Input: part model. Units: mm. Frame: model coordinates. A direction names the side the tool comes from. Give positions to 0.01 mm unless a question says otherwise; leave off trailing zeros. Order: outer loops, then holes, each group sorted by start corner. A loop starts at its lowest first (then second) coordinate and runs counter-clockwise, first axis right, second up. Notation, with made-up numbers: (9.5, -29.75) -> (46.5, -29.75) arc R23 ccw to (46.5, -10.75) -> close; hole circle Ø8 at (43.25, -28.5). An arc over 180 degrees is marked (long way). Use a Markdown table: item, result. Add a question column.
from build123d import *

# Parameters (mm, degrees)
SKETCH1_R                                    = 5
SKETCH1_R_2                                  = 2.5
BOSS_EXTRUDE1_DEPTH                          = 23.5
CSK_FOR_M5_COUNTERSUNK_FLAT_HEAD_SCR_2_COUNT = 2
CSK_FOR_M5_COUNTERSUNK_FLAT_HEAD_SCR_2_PITCH = 25
CUT_EXTRUDE1_DEPTH                           = 31.020826105
CUT_EXTRUDE1_DEPTH_BACK                      = 31.020826105
SKETCH4_W                                    = 10
SKETCH4_H                                    = 11.75


with BuildPart() as part:
    # Sketch1 → Boss-Extrude1 (new, symmetric)
    # profile 1 of 2: a face of its own
    with BuildSketch(Plane.XY):
        with BuildLine():
            Line((-18, -5), (0, -5))
            ThreePointArc((0, -5), (-2.958039892, -4.031128874), (-4.769696007, -1.5))
            Line((-4.769696007, -1.5), (-18, -1.5))
            Line((-18, -1.5), (-18, -5))
        make_face()
    # profile 2 of 2: a face of its own
    with BuildSketch(Plane.XY):
        Circle(SKETCH1_R)
        Circle(SKETCH1_R_2, mode=Mode.SUBTRACT)
    extrude(amount=BOSS_EXTRUDE1_DEPTH, both=True)

    # Sketch3 → CSK for M5 Countersunk Flat Head Screw1 (revolve, cut)
    with BuildSketch(Plane(origin=(-10.5, -1.5, -12.5), x_dir=(0, 0, 1), z_dir=(1, 0, 0))):
        Polygon((0, 0), (0, 3.5), (2.75, 3.5), (2.75, 2.45), (5.2, 0), align=None)
    csk_for_m5_countersunk_flat_head_screw1 = revolve(axis=Axis((-10.5, 4.85, -12.5), (0, -1, 0)), mode=Mode.SUBTRACT)

    # CSK for M5 Countersunk Flat Head Scr 2: CSK for M5 Countersunk Flat Head Screw1 ×2
    with Locations(*[(0, 0, i * CSK_FOR_M5_COUNTERSUNK_FLAT_HEAD_SCR_2_PITCH) for i in range(1, CSK_FOR_M5_COUNTERSUNK_FLAT_HEAD_SCR_2_COUNT)]):
        add(csk_for_m5_countersunk_flat_head_screw1, mode=Mode.SUBTRACT)

    # Sketch4 → Cut-Extrude1 (cut, two sides: drawn at the far end of the back side and taken through both)
    with BuildSketch(Plane(origin=(0, 0, 0), x_dir=(1, 0, 0), z_dir=(0, 1, 0)).offset(-CUT_EXTRUDE1_DEPTH_BACK)):
        with Locations((0, 17.625)):
            Rectangle(SKETCH4_W, SKETCH4_H)
        with Locations((0, -5.875)):
            Rectangle(SKETCH4_W, SKETCH4_H)
    extrude(amount=CUT_EXTRUDE1_DEPTH + CUT_EXTRUDE1_DEPTH_BACK, mode=Mode.SUBTRACT)


solid = part.part
Q1. Access query for faces 4 (the flat face through (-5, -3, 6)), 5 (the cylindrical face through (-13.227, -4.468, 12.142)), 6 (the flat face through (-5, -3, -18)). Directions: +Z, -Z, +X, -X, +Y, -Y. A direction counts if a zero-diameter tool reaches every point of the face in a straight line with its end or side. Return the directions, or none.
Q2. Section query B-B (x = -10.5). Return loops of the section in (y, z).
Q3. Draft query along Y for faces 1 (the flat face through (-9, -5, 0)), 2 (the flat face through (-2, -2, -11.75)), 3 (the cylindrical face through (-0.54, -2.44, 17.54)). Return one class per face: +Y half, -Y half, draft (parallel to the pull), parting line (faces both ways), or undercut.
Q4. Section query D-D (y = 3). Return loops of the section in (x, z), plus the area to 3 significant figures.
Q5. Section query A-A (z = 12.5). Return loops of the section in (x, y), plus the area to 3 significant figures.
Q6. First-contact query: pin 1 (6 mm diameter, centred on x = 0, y = 0, fed in from -Z); pin 2 (1.8 mm diameter, centred on y = -3, z = -17, fed in from +X); pin 3 (2 mm diameter, centred on y = 0, z = 0.5, fed in from -X); pin 4 (8 mm diameter, centred on x = 1, z = 12.5, fed in from +Y). Flat tips, straight axial feed; report the tip coordinate or a pass-through.
Q7. Section query C-C (y = 0). Return loops of the section in (x, z), plus the area to 4 significant figures.
Q8. Ray query, line 1 (Z direction, x = -10.5, y = -4.45); line 2 (Y direction, x = 0, z = 16.75); line 3 (Z direction, x = 4, y = -2.75). Return the intervals inside material, ascending.
Solution:
| question | item | result |
|---|---|---|
| 1 | face 4 | +X, +Y, -Y |
| 1 | face 5 | +Y, -Y |
| 1 | face 6 | -Z, +X, +Y, -Y |
| 2 | outline | (-5, -23.5) -> (-1.5, -23.5) -> (-1.5, -17.7) -> (-3.95, -15.25) -> (-5, -15.25) -> close; (-5, -9.75) -> (-3.95, -9.75) -> (-1.5, -7.3) -> (-1.5, 7.3) -> (-3.95, 9.75) -> (-5, 9.75) -> close; (-5, 15.25) -> (-3.95, 15.25) -> (-1.5, 17.7) -> (-1.5, 23.5) -> (-5, 23.5) -> close |
| 3 | face 1 | -Y half |
| 3 | face 2 | draft |
| 3 | face 3 | undercut |
| 4 | outline | (-4, -11.75) -> (4, -11.75) -> (4, 0) -> (-4, 0) -> close; (-4, 11.75) -> (4, 11.75) -> (4, 23.5) -> (-4, 23.5) -> close |
| 4 | area | 188 mm² |
| 5 | outline | (-18, -5) -> (-13.25, -5) -> (-13.25, -3.95) -> (-15.7, -1.5) -> (-18, -1.5) -> close; (-7.75, -5) -> (0, -5) arc R5 ccw (long way) to (-4.77, -1.5) -> (-5.3, -1.5) -> (-7.75, -3.95) -> close; hole circle Ø5 at (0, 0) |
| 5 | area | 84.4 mm² |
| 6 | pin 1 | stops at z = -11.75 |
| 6 | pin 2 | stops at x = -5 |
| 6 | pin 3 | stops at x = -5 |
| 6 | pin 4 | stops at y = 5 |
| 7 | outline | (-5, -11.75) -> (-2.5, -11.75) -> (-2.5, 0) -> (-5, 0) -> close; (-5, 11.75) -> (-2.5, 11.75) -> (-2.5, 23.5) -> (-5, 23.5) -> close; (2.5, -11.75) -> (5, -11.75) -> (5, 0) -> (2.5, 0) -> close; (2.5, 11.75) -> (5, 11.75) -> (5, 23.5) -> (2.5, 23.5) -> close |
| 7 | area | 117.5 mm² |
| 8 | line 1 | z = -23.5 to -15.25, -9.75 to 9.75, 15.25 to 23.5 |
| 8 | line 2 | y = -5 to -2.5, 2.5 to 5 |
| 8 | line 3 | z = -11.75 to 0, 11.75 to 23.5 |
